Geometry: final body of the model. Coordinates: model frame, mm. A direction names the side the tool comes from. Coordinates: 2 decimals unless noted, no trailing zeros. Write each loop counter-clockwise with the first axis right and the second up, starting at its lowest first coordinate (ties: lowest second). Pieces come first, ordered by that corner, then holes. Notation, with made-up numbers: M 8,17.25 L 59,17.25 A22 ccw 59,26.25 Z; hole C -1,-31 d9. An arc over 180 degrees is marked long. Write item = value, one per line. Start each with the question number.
Item 1: Ray query, L1, parallel to X at y = -17, z = 64.5; L2, parallel to Z at x = 0, y = -20 (3 decimals); L3, parallel to Z at x = -21, y = 29.5. Return the intervals inside material, ascending. Write a range as [from, to].
Item 2: First-contact query: pin 1 Ø11 at (x, y) = (-25.49, -39.47) entering from +Z; pin 2 Ø15 at (x, z) = (-14.5, 54.5) entering from +Y; pin 3 Ø6 at (x, y) = (0, -1.5) entering from +Z (3 decimals); pin 4 Ø11 at (x, y) = (25.56, 31.49) entering from -Z. Flat tips, straight axial feed; report the tip coordinate or a pass-through.
Item 3: Reachability of faces 4 (the flat face through (1, -39, 19.05)), 5 (the cylindrical face through (-20.868, 31.279, 9.658)), 6 (the flat face through (-1, 0, 39)), 7 (the flat face through (0, -13, 41.275)), 8 (the flat face through (38.1, -5, 20)) from +Z, -Z, +X, -X, +Y, -Y: full face, straight path, thin tool, end or side. Return the list, or none.
Item 4: Section A-A on z = 46.5. Output: boundary loops of the cut face in (x, y).
Item 5: Section C-C on y = -36. Output: boundary loops of the cut face in (x, z), plus the area to 3 significant figures.
Item 6: Pull-direction query (X, two-part tool) for faces 1 (the cylindrical face through (22.97, -43.44, 9.66)), 2 (the flat face through (1, 23, 19.05)), 3 (the flat face through (-38.1, -5, 20)); classes: +X half, -X half, draft (parallel to the pull), parting line (faces both ways), or undercut.
Item 7: Section D-D on x = 23. Output: boundary loops of the cut face in (y, z), plus the area to 3 significant figures.
Item 8: Section B-B on x = 11. Output: boundary loops of the cut face in (y, z) (3 decimals).
from build123d import *

# Parameters (mm, degrees)
F1_DEPTH = 25.4
F3_DEPTH = 38.1
F5_D     = 9.398


with BuildPart() as f1:
    # F0 (on Front) → F1 (new body)
    with BuildSketch(Plane.XZ):
        Polygon((-38.1, 0), (38.1, 0), (38.1, 69.85), (14.5568246901, 69.85), (14.5568246901, 41.275), (-14.2748, 41.275), (-14.2748, 69.85), (-38.1, 69.85), align=None)
    extrude(amount=F1_DEPTH)

    # F2 (on Right) → F3 (join, symmetric)
    with BuildSketch(Plane.YZ):
        Polygon((-52.1549474458, 0), (0, 0), (43.0950525542, 0), (44.45, 19.05), (0, 19.05), (-52.1549474458, 19.05), align=None)
    extrude(amount=F3_DEPTH, both=True)

    # F5 (through all)
    with Locations(Plane(origin=(0, 0, 0), x_dir=(1, 0, 0), z_dir=(0, 0, -1))):
        with Locations((-25.4933413446, 39.4742776036), (25.4933413446, 39.4742776036), (25.5620578019, -31.4856089659), (-25.5620578019, -31.4856089659)):
            Hole(F5_D / 2)


solid = f1.part
Responses:
q1.L1 = [-38.1, -14.27], [14.56, 38.1]
q1.L2 = [0, 41.275]
q1.L3 = [0, 19.05]
q2.pin_1 = 19.05
q2.pin_2 = 0
q2.pin_3 = 41.275
q2.pin_4 = 0
q3.face_4 = +Z, +X, -X, -Y
q3.face_5 = +Z, -Z
q3.face_6 = +Z, +X, -X, +Y
q3.face_7 = +Z, +Y, -Y
q3.face_8 = +Z, -Z, +X, +Y, -Y
q4.outline = M -38.1,-25.4 L -14.27,-25.4 L -14.27,0 L -38.1,0 Z; M 14.56,-25.4 L 38.1,-25.4 L 38.1,0 L 14.56,0 Z
q5.outline = M -38.1,0 L -28.66,0 L -28.66,19.05 L -38.1,19.05 Z; M -22.33,0 L 22.33,0 L 22.33,19.05 L -22.33,19.05 Z; M 28.66,0 L 38.1,0 L 38.1,19.05 L 28.66,19.05 Z
q5.area = 1,210 mm²
q6.face_1 = undercut
q6.face_2 = draft
q6.face_3 = -X half
q7.outline = M -52.15,0 L -43.46,0 L -43.46,19.05 L -52.15,19.05 Z; M -35.49,0 L 27.55,0 L 27.55,19.05 L 0,19.05 L 0,69.85 L -25.4,69.85 L -25.4,19.05 L -35.49,19.05 Z; M 35.42,0 L 43.1,0 L 44.45,19.05 L 35.42,19.05 Z
q7.area = 2,820 mm²
q8.outline = M -52.155,0 L 43.095,0 L 44.45,19.05 L 0,19.05 L 0,41.275 L -25.4,41.275 L -25.4,19.05 L -52.155,19.05 Z
